For this review, take the finished solid that the model builds, in its own axes (mm). Coordinates: 2 decimals unless noted, no trailing zeros. Loops run counter-clockwise (first coordinate to the right, second up) from the corner with the lowest first, then second, coordinate; pieces in that order, holes last.
1. Take a section at C-C, the plane z = 0. State the section outline as (x, y) points.
2. To check wall thickness, follow probe 1 along Z at (x, y) = (45, -2.75); probe 2 along Z at (x, y) = (173.5, -8.25); probe 3 along X at (y, z) = (-5.75, 5.5). State the ranges of each line that lie inside material, in increasing order.
3. Take a section at B-B, the plane y = -6.5. State the section outline as (x, z) points.
4. Take a section at A-A, the plane x = 57.5. State the section outline as (y, z) points.
5. Take a section at D-D, the plane x = -141. State the section outline as (y, z) points.
6. Clearance check with flat-ended pins moving along their axes: P1, Ø6, axis at y = -9, z = -122, coming from the -X side; P2, Ø3, axis at x = 20.5, y = -10.5, coming from the +Z side; P3, Ø6, axis at x = -124.5, y = -8, coming from the +Z side; P4, Ø4, axis at x = 36.5, z = -148, coming from the +Y side. State where each tip first meets the part, or that it passes through.
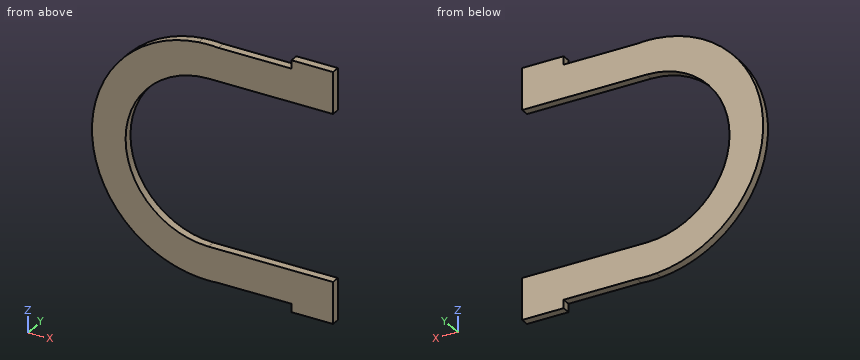
```python
from build123d import *

# Parameters (mm, degrees)
F1_DEPTH = 12.7


with BuildPart() as f1:
    # F0 (on Front) → F1 (new body)
    with BuildSketch(Plane.XZ):
        with BuildLine():
            Line((127, 190.5), (127, 177.8))
            Line((127, 177.8), (15.045787, 177.8))
            Line((15.045787, 177.8), (-15.045787, 177.8))
            ThreePointArc((-15.045787, 177.8), (-178.435466, 0), (-15.045787, -177.8))
            Line((-15.045787, -177.8), (15.045787, -177.8))
            Line((15.045787, -177.8), (127, -177.8))
            Line((127, -177.8), (127, -190.5))
            Line((127, -190.5), (190.5, -190.5))
            Line((190.5, -190.5), (190.5, -177.8))
            Line((190.5, -177.8), (190.5, -127))
            Line((190.5, -127), (127, -127))
            Line((127, -127), (0, -127))
            ThreePointArc((0, -127), (-127, 0), (0, 127))
            Line((0, 127), (127, 127))
            Line((127, 127), (190.5, 127))
            Line((190.5, 127), (190.5, 177.8))
            Line((190.5, 177.8), (190.5, 190.5))
            Line((190.5, 190.5), (127, 190.5))
        make_face()
        with BuildLine():
            Line((-15.045787, 177.8), (15.045787, 177.8))
            ThreePointArc((15.045787, 177.8), (0, 178.435466), (-15.045787, 177.8))
        make_face()
        with BuildLine():
            Line((15.045787, -177.8), (-15.045787, -177.8))
            ThreePointArc((-15.045787, -177.8), (0, -178.435466), (15.045787, -177.8))
        make_face()
    extrude(amount=F1_DEPTH)


solid = f1.part
```
Results list:
1. outline: (-178.44, -12.7) - (-127, -12.7) - (-127, 0) - (-178.44, 0) - close
2. probe 1: z = -177.8 to -127, 127 to 177.8
2. probe 2: z = -190.5 to -127, 127 to 190.5
2. probe 3: x = -178.35 to -126.88
3. outline: (-15.05, -177.8) arc R178.44 ccw to (15.05, -177.8) - (127, -177.8) - (127, -190.5) - (190.5, -190.5) - (190.5, -127) - (0, -127) arc R127 cw to (0, 127) - (190.5, 127) - (190.5, 190.5) - (127, 190.5) - (127, 177.8) - (15.05, 177.8) arc R178.44 ccw to (-15.05, 177.8) arc R178.44 ccw to start
4. outline: (-12.7, -177.8) - (0, -177.8) - (0, -127) - (-12.7, -127) - close; (-12.7, 127) - (0, 127) - (0, 177.8) - (-12.7, 177.8) - close
5. outline: (-12.7, -109.35) - (0, -109.35) - (0, 109.35) - (-12.7, 109.35) - close
6. P1: stops at x = -132.96
6. P2: stops at z = 177.8
6. P3: stops at z = 130.68
6. P4: stops at y = 0
